Verification items for the finished model (mm, model axes). A direction names the side the tool comes from. Give positions to 0.01 mm unless a question says otherwise; leave off trailing zeros. Write each loop counter-clockwise with the first axis right and the second up, starting at its lowest first coordinate (ties: lowest second). Pieces come first, ordered by that corner, then holes.
Autodesk Inventor part; units mm, degrees
ref_plane "YZ Plane" through (0, 0, 0) normal (1, 0, 0) x (0, 1, 0)
ref_plane "XZ Plane" through (0, 0, 0) normal (0, 1, 0) x (-1, 0, 0)
ref_plane "XY Plane" through (0, 0, 0) normal (0, 0, 1) x (1, 0, 0)
sketch "Sketch1" plane through (0, 0, 0) normal (0, 0, 1) x (1, 0, 0)
  line L0 (0, 0) -> (80, 0)
  line L1 (80, 0) -> (80, 10)
  line L2 (80, 10) -> (50, 10)
  line L3 (50, 10) -> (50, 50)
  line L4 (50, 50) -> (30, 50)
  line L5 (30, 50) -> (30, 10)
  line L6 (30, 10) -> (0, 10)
  line L7 (0, 10) -> (0, 0)
  dimension "d0" = 80
  dimension "d1" = 10
  dimension "d2" = 40
extrude "Extrusion1" add sketch "Sketch1" along normal blind 60
sketch "Sketch2" plane through (50, 10, 0) normal (1, 0, 0) x (0, 0, -1)
  line L0 (-10, 10) -> (-25, 10)
  line L1 (-25, 10) -> (-25, 30)
  line L2 (-25, 30) -> (-10, 30)
  line L3 (-10, 30) -> (-10, 10)
  line L4 (-50, 30) -> (-50, 10)
  line L5 (-50, 10) -> (-35, 10)
  line L6 (-35, 10) -> (-35, 30)
  line L7 (-35, 30) -> (-50, 30)
  point P0 (0, -10)
extrude "Extrusion2" add sketch "Sketch2" along normal blind 25 contours L0 L1 L2 L3
sketch "Sketch3" plane through (50, 10, 0) normal (1, 0, 0) x (0, 0, -1)
  line L0 (-35, 30) -> (-35, 10)
  line L1 (-35, 10) -> (-50, 10)
  line L2 (-50, 10) -> (-50, 30)
  line L3 (-60, 40) -> (-60, 0)
  line L4 (-50, 30) -> (-35, 30)
  point P0 (0, -10)
extrude "Extrusion3" cut sketch "Sketch3" against normal blind 20
properties part number "P3-8"
Item 1: Sectioned sample at A-A on y = 36. Record the cut outline in (x, z), then the cut area to 4 significant figures.
Answer key:
outline: (30, 0) - (50, 0) - (50, 10) - (75, 10) - (75, 25) - (50, 25) - (50, 35) - (30, 35) - close; (30, 50) - (50, 50) - (50, 60) - (30, 60) - close
area: 1,275 mm2
Item 2: Sectioned sample at D-D on x = 42.5. Record the cut outline in (y, z), then the cut area to 3 significant figures.
Answer key:
outline: (0, 0) - (50, 0) - (50, 60) - (0, 60) - close; hole (20, 35) - (40, 35) - (40, 50) - (20, 50) - close
area: 2,700 mm2
Item 3: Sectioned sample at B-B on x = 51. Record the cut outline in (y, z), then the cut area to 3 significant figures.
Answer key:
outline: (0, 0) - (10, 0) - (10, 60) - (0, 60) - close; (20, 10) - (40, 10) - (40, 25) - (20, 25) - close
area: 900 mm2
Item 4: Sectioned sample at C-C on z = 37. Record the cut outline in (x, y).
Answer key:
outline: (0, 0) - (80, 0) - (80, 10) - (50, 10) - (50, 20) - (30, 20) - (30, 10) - (0, 10) - close; (30, 40) - (50, 40) - (50, 50) - (30, 50) - close
Item 5: Scan lines: line 1 along Y through (x, z) = (74.5, 17.5); line 2 along Z through (x, y) = (34, 22.5); line 3 along X through (y, z) = (42, 12.5). Record each from-to range of solid material in increasing order.
Answer key:
line 1: y = 0 to 10, 20 to 40
line 2: z = 0 to 35, 50 to 60
line 3: x = 30 to 50
Item 6: Set-up check for faces 4 (the face through (75, 30, 18)), 5 (the face through (62, 20, 17)), 6 (the face through (62, 30, 10)), 7 (the face through (40, 30, 35)): record each of +Z, -Z, +X, -X, +Y, -Y from which the full face is reachable in a straight line by a thin tool's end or side.
Answer key:
face 4: +Z, -Z, +X, +Y
face 5: +Z, -Z, +X
face 6: -Z, +X, +Y
face 7: +X, -X
Item 7: Depth check by flat-ended pin: pin 1 (16.5 mm diameter, centred on y = 34.5, z = 16, fed in from +X); pin 2 (15 mm diameter, centred on x = 68, z = 18.5, fed in from +Y); pin 3 (12 mm diameter, centred on y = 35.5, z = 37, fed in from -X). Enter the tip coordinate at first touch or a pass-through.
Answer key:
pin 1: stops at x = 75
pin 2: stops at y = 40
pin 3: stops at x = 30
Item 8: Release check for a two-part mould opening along Y. For faces 1 (the face through (80, 5, 30)), 2 (the face through (65, 10, 30)), 3 (the face through (62, 40, 18)) record: released by +Y, released by -Y, zero draft, split by the parting line, or undercut.
Answer key:
face 1: zero draft
face 2: undercut
face 3: released by +Y
